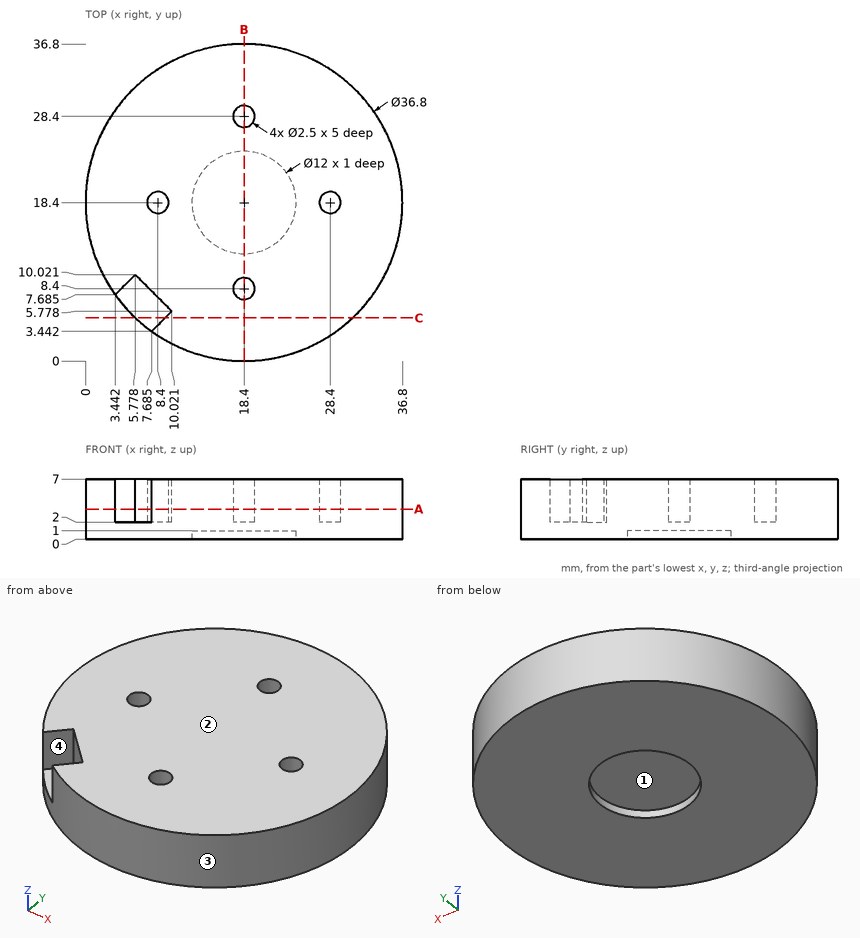
Study the drawing (mm; zero at the part's minimum x, y, z) and answer. Round coordinates to 2 decimals unless told otherwise and drop trailing zeros. Write each loop counter-clockwise with the first axis right and the second up, starting at its lowest first coordinate (ties: lowest second). Pieces come first, ordered by that corner, then holes. Notation, with made-up numbers: (-24.75, -36.75) - (-9.75, -36.75) arc R17 cw to (-9.75, -3.75) - close; hole circle Ø6 at (39.25, -18). An arc over 180 degrees is marked (long way). Return JSON: item names as keys, results as strings. Group by question number.
Q1. Find the intervals of material crossed by L1, parallel to Y at x = 18.4, z = 3.9; L2, parallel to X at y = 18, z = 3.75 (1 decimal); L3, parallel to X at y = 19.5, z = 2.5 (1 decimal), in increasing order.
Q2. Each of these flat-tipped pins is pushed along its axis until it touches: pin 1 Ø1.2 at (x, y) = (19, 28.5) entering from +Z; pin 2 Ø2 at (x, z) = (10.5, 6) entering from -Y; pin 3 Ø4 at (x, z) = (11, 1) entering from +Y. Where does it stop, or does it pass through?
Q3. The part is cut by section B-B on x = 18.4. Write down the section's boundary in (y, z).
Q4. The part is cut by section C-C on y = 5. Write down the section's boundary in (x, z).
Q5. The mould has two halves that part along Y. Classify the marked faces 1, 2, 3 and 4: released by +Y, released by -Y, zero draft, split by the parting line, or undercut.
Q6. The part is cut by section A-A on z = 3.5. Count the separate pieces of the cut face and the enclosed holes in it, then the cut area to 3 significant figures.
Solved:
{
 "1": {"L1": "0 to 7.15, 9.65 to 27.15, 29.65 to 36.8", "L2": "0 to 7.2, 9.6 to 27.2, 29.6 to 36.8", "L3": "0 to 7.8, 9 to 27.8, 29 to 36.8"},
 "2": {"pin 1": "z = 2", "pin 2": "y = 1.34", "pin 3": "y = 35.99"},
 "3": {"outline": "(0, 0) - (12.4, 0) - (12.4, 1) - (24.4, 1) - (24.4, 0) - (36.8, 0) - (36.8, 7) - (29.65, 7) - (29.65, 2) - (27.15, 2) - (27.15, 7) - (9.65, 7) - (9.65, 2) - (7.15, 2) - (7.15, 7) - (0, 7) - close"},
 "4": {"outline": "(5.79, 0) - (31.01, 0) - (31.01, 7) - (9.24, 7) - (9.24, 2) - (5.79, 2) - close"},
 "5": {"face 1": "undercut", "face 2": "zero draft", "face 3": "split by the parting line", "face 4": "released by -Y"},
 "6": {"separate pieces": "1", "enclosed holes": "4", "area": "1,020 mm²"}
}
